```python
from build123d import *

# Parameters (mm, degrees)
BOSS_EXTRUDE1_DEPTH = 5.9944
SKETCH2_R           = 5.08
CUT_EXTRUDE1_DEPTH  = 390.227437664
CUT_EXTRUDE2_DEPTH  = 1.27
FILLET1_R           = 6.35


with BuildPart() as part:
    # Sketch1 → Boss-Extrude1 (new body)
    with BuildSketch(Plane(origin=(0, 0, 0), x_dir=(1, 0, 0), z_dir=(0, 1, 0))):
        Polygon((-60.325, 0), (62.865, 0), (158.147732829, -355.6), (-155.607732829, -355.6), align=None)
    extrude(amount=BOSS_EXTRUDE1_DEPTH)

    # Sketch2 → Cut-Extrude1 (cut, through all)
    with BuildSketch(Plane(origin=(0, 5.9944, 0), x_dir=(1, 0, 0), z_dir=(0, 1, 0))):
        with Locations(Location((1.27, -101.6, 0), (0, 0, 270))):
            Circle(SKETCH2_R)
    extrude(amount=-CUT_EXTRUDE1_DEPTH, mode=Mode.SUBTRACT)

    # Sketch3 → Cut-Extrude2 (cut)
    with BuildSketch(Plane(origin=(0, 5.9944, 0), x_dir=(1, 0, 0), z_dir=(0, 1, 0))):
        with BuildLine():
            Line((-2.004607843, -124.878144621), (-2.801470588, -124.878144621))
            Line((-2.801470588, -124.878144621), (-2.801470588, -116.532875013))
            add(Edge.make_bspline(
                [(-2.801470588, -116.532875013), (-2.997580196, -116.700819797), (-3.386189924, -117.033618267), (-4.021446732, -117.460305556), (-4.686888668, -117.826576867), (-5.156638111, -118.012129239), (-5.39127451, -118.104811287)],
                knots=[0, 0, 0, 0, 1.01587232, 2.013047047, 3.007531584, 4, 4, 4, 4], degree=3))
            Line((-5.39127451, -118.104811287), (-5.39127451, -117.307948542))
            add(Edge.make_bspline(
                [(-5.39127451, -117.307948542), (-5.215920906, -117.217505842), (-4.877167455, -117.042785871), (-4.403316888, -116.758839494), (-3.978244692, -116.470049726), (-3.602949198, -116.17444242), (-3.276786637, -115.872526552), (-3.001240232, -115.563383013), (-2.771725814, -115.249055295), (-2.657674184, -115.025829059), (-2.602254902, -114.917360307)],
                knots=[0, 0, 0, 0, 1.266365021, 2.446402654, 3.543839948, 4.563310278, 5.51059178, 6.392882026, 7.219078889, 8, 8, 8, 8], degree=3))
            Line((-2.602254902, -114.917360307), (-2.004607843, -114.917360307))
            Line((-2.004607843, -114.917360307), (-2.004607843, -124.878144621))
        make_face()
        with BuildLine():
            Line((7.756960784, -124.878144621), (1.382058824, -124.878144621))
            add(Edge.make_bspline(
                [(1.382058824, -124.878144621), (1.408711728, -124.714616011), (1.461765394, -124.389105805), (1.581972244, -123.981996467), (1.743426669, -123.650686593), (1.9293472, -123.370987394), (2.168929241, -123.057519518), (2.47120082, -122.71410621), (2.835292405, -122.341606598), (3.26682725, -121.943231351), (3.76528863, -121.520849044), (4.12547647, -121.238121937), (4.314264706, -121.089933836)],
                knots=[0, 0, 0, 0, 1.00794059, 2.006345856, 2.568221262, 3.244176762, 4.045978883, 4.967707078, 6.025786227, 7.214078669, 8.539791974, 10, 10, 10, 10], degree=3))
            add(Edge.make_bspline(
                [(4.314264706, -121.089933836), (4.44517426, -120.987435642), (4.692315869, -120.79393129), (5.03663113, -120.518956984), (5.330891728, -120.274531461), (5.654603916, -119.998078646), (6.00245485, -119.669813627), (6.353952481, -119.268109359), (6.634490533, -118.868145818), (6.82961898, -118.465238329), (6.941715143, -118.053908101), (6.953924697, -117.775536057), (6.960098039, -117.634786777)],
                knots=[0, 0, 0, 0, 1.105083233, 2.086265203, 2.928643677, 3.647492745, 4.915719202, 6.103603942, 7.190110835, 8.152548768, 9.065899631, 10, 10, 10, 10], degree=3))
            add(Edge.make_bspline(
                [(6.960098039, -117.634786777), (6.956446087, -117.531840775), (6.949349268, -117.331786414), (6.896203587, -117.042256181), (6.805514931, -116.774954845), (6.678536736, -116.530021827), (6.524513793, -116.305351489), (6.336809674, -116.107371083), (6.124267579, -115.931524187), (5.883239638, -115.782669248), (5.619825862, -115.659684087), (5.331783261, -115.577707036), (5.025139044, -115.521422364), (4.812576912, -115.517184746), (4.703357843, -115.515007366)],
                knots=[0, 0, 0, 0, 1.066440105, 2.072406788, 3.038089023, 3.980626898, 4.923164774, 5.851240192, 6.79842777, 7.774055624, 8.779619978, 9.800248095, 10.869719403, 12, 12, 12, 12], degree=3))
            add(Edge.make_bspline(
                [(4.703357843, -115.515007366), (4.548138853, -115.520928959), (4.250554949, -115.532281765), (3.828569287, -115.636647969), (3.455686954, -115.810346784), (3.131253079, -116.053703201), (2.863324958, -116.371844332), (2.643875434, -116.754056503), (2.47967465, -117.206553497), (2.413141707, -117.534067539), (2.378137255, -117.706379915)],
                knots=[0, 0, 0, 0, 1.052503955, 2.0178474, 2.928593632, 3.828899676, 4.748107049, 5.732867451, 6.807211463, 8, 8, 8, 8], degree=3))
            Line((2.378137255, -117.706379915), (1.58127451, -117.581870111))
            add(Edge.make_bspline(
                [(1.58127451, -117.581870111), (1.595076615, -117.472635137), (1.622075599, -117.258955176), (1.691468745, -116.949821561), (1.781188383, -116.65900971), (1.894180859, -116.386211747), (2.027180985, -116.131787712), (2.181450374, -115.894298832), (2.359285462, -115.67667965), (2.558282869, -115.477221584), (2.777101916, -115.300105787), (3.010614318, -115.143004122), (3.261947111, -115.012623851), (3.527029837, -114.902576084), (3.808744154, -114.818752319), (4.105725503, -114.759825606), (4.418264758, -114.725756279), (4.631681691, -114.72071836), (4.740710784, -114.718144621)],
                knots=[0, 0, 0, 0, 1.11558569, 2.182252598, 3.206865404, 4.197163727, 5.171016007, 6.113287932, 7.062752653, 8.014719109, 8.96418383, 9.912249364, 10.862587531, 11.829428462, 12.817713982, 13.836697005, 14.894825442, 16, 16, 16, 16], degree=3))
            add(Edge.make_bspline(
                [(4.740710784, -114.718144621), (4.847691173, -114.72046441), (5.058171976, -114.725028527), (5.36652187, -114.763086832), (5.660393604, -114.82495492), (5.939114933, -114.911807601), (6.20152099, -115.026029366), (6.453209418, -115.158232899), (6.686929332, -115.3230483), (6.90677244, -115.507442597), (7.10466303, -115.712898212), (7.281765919, -115.930826025), (7.427856103, -116.167038419), (7.551242282, -116.415109275), (7.639716311, -116.6810721), (7.709539512, -116.957384709), (7.75083418, -117.249641754), (7.754889172, -117.448930261), (7.756960784, -117.55074266)],
                knots=[0, 0, 0, 0, 1.106681904, 2.177364475, 3.209175827, 4.210887483, 5.192078542, 6.167200624, 7.147039734, 8.145062256, 9.132109826, 10.094560107, 11.044836899, 12.000375742, 12.954465884, 13.938765234, 14.946957558, 16, 16, 16, 16], degree=3))
            add(Edge.make_bspline(
                [(7.756960784, -117.55074266), (7.753392459, -117.673373377), (7.746338565, -117.915790814), (7.689282598, -118.27439108), (7.590587318, -118.620687231), (7.461036956, -118.958802553), (7.290519429, -119.282309345), (7.09006167, -119.596153204), (6.8567572, -119.897227952), (6.634069689, -120.13817633), (6.430892234, -120.330451922), (6.256380071, -120.493260828), (6.057657341, -120.670326555), (5.833743473, -120.859320414), (5.585765126, -121.061219336), (5.319829881, -121.283578823), (5.026752033, -121.516537042), (4.821857186, -121.674370634), (4.715808824, -121.756061287)],
                knots=[0, 0, 0, 0, 1.088993338, 2.152731221, 3.214950677, 4.282992305, 5.363056107, 6.45734114, 7.587448717, 8.741912054, 9.367708333, 10.072059012, 10.861970471, 11.731730561, 12.674646287, 13.702521352, 14.810883478, 16, 16, 16, 16], degree=3))
            add(Edge.make_bspline(
                [(4.715808824, -121.756061287), (4.589531577, -121.855817691), (4.343139397, -122.050462401), (3.994847151, -122.350096885), (3.673432745, -122.643330902), (3.386447313, -122.938064959), (3.127000006, -123.22720294), (2.897403274, -123.51287463), (2.693792631, -123.79321546), (2.582015901, -123.986901831), (2.52754902, -124.081281875)],
                knots=[0, 0, 0, 0, 1.201760701, 2.344875646, 3.430713183, 4.449969728, 5.415927222, 6.330865599, 7.186659457, 8, 8, 8, 8], degree=3))
            Line((2.52754902, -124.081281875), (7.756960784, -124.081281875))
            Line((7.756960784, -124.081281875), (7.756960784, -124.878144621))
        make_face()
    extrude(amount=-CUT_EXTRUDE2_DEPTH, mode=Mode.SUBTRACT)

    # Fillet1
    fillet1_edges = [part.edges().sort_by_distance(p)[0] for p in [
        (158.147732829, 2.9972, 355.6),
        (-155.607732829, 2.9972, 355.6),
        (-60.325, 2.9972, 0),
        (62.865, 2.9972, 0),
    ]]
    fillet(fillet1_edges, radius=FILLET1_R)


solid = part.part
```
CAD build for the part. Positions are in the model's coordinates, mm. Round coordinates to 2 decimals unless told otherwise and drop trailing zeros. Loops run counter-clockwise (first coordinate to the right, second up) from the corner with the lowest first, then second, coordinate; pieces in that order, holes last. Notation, with made-up numbers: M 33.5,16 L 72.5,16 A19 cw 72.5,50 Z; hole C -15.5,54 d10. An arc over 180 degrees is marked long. Return JSON: item names as keys, results as strings. Group by question number.
(1) Mould opens along X. For faces 1 (the flat face through (109.423, 2.955, 173.756)), 2 (the flat face through (3, 5.994, 215)), 3 (the cylindrical face through (2.796, 3.039, 106.445)) say: +X half, -X half, draft (parallel to the pull), parting line (faces both ways), or undercut.
(2) Drop flat-ended pins along their axis: P1, Ø1, axis at y = 0.5, z = 210, coming from the +X side; P2, Ø2, axis at y = 3, z = 270.5, coming from the +X side. Give the stop position or say it passes through.
(3) Saw through at B-B, the plane z = 101.6. List the corners of the cut face in (x, y).
(4) Saw through at A-A, the plane y = 3.8. List the corners of the cut face in (x, z), and give its area (3 significant figures).
(5) Saw through at C-C, the plane x = -129. List the corners of the cut face in (y, z).
(6) Saw through at D-D, the plane z = 182.5. List the corners of the cut face in (x, y).
(7) Wall check: probe 1 along X at (y, z) = (3.1, 101.6); probe 2 along Z at (x, y) = (4, 1.35); probe 3 along X at (y, z) = (4.05, 109.5). Give the ranges that are in metal, low to high. Write a range as [from, to].
Answer list:
{
 "1": {"face 1": "+X half", "face 2": "draft", "face 3": "undercut"},
 "2": {"P1": "x = 119.27", "P2": "x = 135.61"},
 "3": {"outline": "M -87.55,0 L -3.81,0 L -3.81,5.99 L -87.55,5.99 Z; M 6.35,0 L 90.09,0 L 90.09,5.99 L 6.35,5.99 Z"},
 "4": {"outline": "M -153.47,347.61 L -61.59,4.71 A6.35 ccw -55.45,0 L 57.99,0 A6.35 ccw 64.13,4.71 L 156.01,347.61 A6.35 ccw 149.87,355.6 L -147.33,355.6 A6.35 ccw Z; hole C 1.27,101.6 d10.16", "area": "77,600 mm2"},
 "5": {"outline": "M 0,256.3 L 5.99,256.3 L 5.99,355.6 L 0,355.6 Z"},
 "6": {"outline": "M -109.23,0 L 111.77,0 L 111.77,5.99 L -109.23,5.99 Z"},
 "7": {"probe 1": "[-87.55, -3.81], [6.35, 90.09]", "probe 2": "[0, 97.32], [105.88, 355.6]", "probe 3": "[-89.67, 92.21]"}
}
